Could you check a few things on this model? Use its own coordinates, in mm. Face numbers are marked on the shaded views. A direction names the side the tool comes from. Give positions to 0.01 mm unless a question says otherwise; leave off trailing zeros.
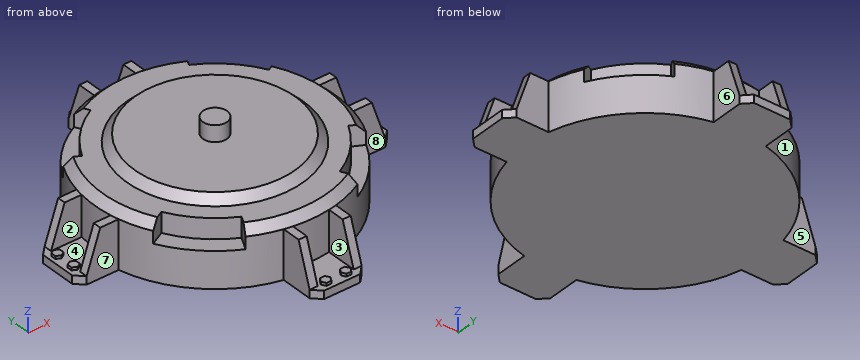
from build123d import *

# Parameters (mm, degrees)
SKETCH1_R                    = 150
BOSS_EXTRUDE1_DEPTH          = 70
CHAMFER1_SIZE                = 10
BOSS_EXTRUDE2_START          = -70
BOSS_EXTRUDE2_DEPTH          = 10
CHAMFER2_SIZE                = 10
BOSS_EXTRUDE3_DEPTH          = 10
BOSS_EXTRUDE4_DEPTH          = 3.5
CIRPATTERN1_COUNT            = 4
CIRPATTERN1_COPY_1_DEPTH     = 10
CIRPATTERN1_COPY_2_DEPTH     = 10
CIRPATTERN1_COPY_3_DEPTH     = 10
CIRPATTERN1_COPY_4_DEPTH     = 3.5
CIRPATTERN1_COPY_5_DEPTH     = 3.5
CIRPATTERN1_COPY_6_DEPTH     = 3.5
CHAMFER2_OF_CIRPATTERN1_SIZE = 10
CUT_EXTRUDE1_START           = -25
CUT_EXTRUDE1_DEPTH           = 25
CIRPATTERN2_COUNT            = 4
SKETCH6_R                    = 110
BOSS_EXTRUDE5_DEPTH          = 10
CHAMFER3_SIZE                = 10
SKETCH8_R                    = 15
BOSS_EXTRUDE6_DEPTH          = 20
BODY_MOVE_COPY2_ANGLE        = 90


with BuildPart() as part:
    # Sketch1 → Boss-Extrude1 (new body)
    with BuildSketch(Plane(origin=(0, 0, 0), x_dir=(1, 0, 0), z_dir=(0, 1, 0))):
        with Locations(Location((0, 0, 0), (0, 0, 270))):
            Circle(SKETCH1_R)
    extrude(amount=BOSS_EXTRUDE1_DEPTH)

    # Chamfer1
    chamfer1_edges = [part.edges().sort_by_distance(p)[0] for p in [
        (0, 70, -150),
    ]]
    chamfer(chamfer1_edges, length=CHAMFER1_SIZE)

    # Sketch2 → Boss-Extrude2 (add)
    with BuildSketch(Plane(origin=(0, 70, 0), x_dir=(1, 0, 0), z_dir=(0, 1, 0)).offset(BOSS_EXTRUDE2_START)):
        with BuildLine():
            Line((-146.436846456, 32.5), (-196.436846456, 32.5))
            Line((-196.436846456, 32.5), (-196.436846456, -32.5))
            Line((-196.436846456, -32.5), (-146.436846456, -32.5))
            ThreePointArc((-146.436846456, -32.5), (-150, 0), (-146.436846456, 32.5))
        make_face()
    boss_extrude2 = extrude(amount=BOSS_EXTRUDE2_DEPTH)

    # Chamfer2
    chamfer2_edges = [part.edges().sort_by_distance(p)[0] for p in [
        (-196.436846456, 5, -32.5),
        (-196.436846456, 5, 32.5),
    ]]
    chamfer(chamfer2_edges, length=CHAMFER2_SIZE)

    # Sketch3 → Boss-Extrude3 (add)
    with BuildSketch(Plane.XY.offset(32.5)):
        Polygon((-146.436846456, 10), (-146.436846456, 60), (-169.436846456, 60), (-186.436846456, 10), align=None)
    boss_extrude3 = extrude(amount=-BOSS_EXTRUDE3_DEPTH)

    # Sketch4 → Boss-Extrude4 (add)
    with BuildSketch(Plane(origin=(0, 10, 0), x_dir=(1, 0, 0), z_dir=(0, 1, 0))):
        Polygon((-186.436846456, -6.5), (-191.632998879, -9.5), (-191.632998879, -15.5), (-186.436846456, -18.5), (-181.240694033, -15.5), (-181.240694033, -9.5), align=None)
    boss_extrude4 = extrude(amount=BOSS_EXTRUDE4_DEPTH)

    # Mirror1: Boss-Extrude3, Boss-Extrude4 across plane
    add(boss_extrude3.mirror(Plane.XY))
    add(boss_extrude4.mirror(Plane.XY))

    # CirPattern1: Boss-Extrude2, Boss-Extrude3, Boss-Extrude4 ×4 about axis
    cirpattern1_axis = Axis((0, 0, 0), (0, 1, 0))
    add([boss_extrude2.rotate(cirpattern1_axis, i * 360 / CIRPATTERN1_COUNT) for i in range(1, CIRPATTERN1_COUNT)])
    add([boss_extrude3.rotate(cirpattern1_axis, i * 360 / CIRPATTERN1_COUNT) for i in range(1, CIRPATTERN1_COUNT)])
    add([boss_extrude4.rotate(cirpattern1_axis, i * 360 / CIRPATTERN1_COUNT) for i in range(1, CIRPATTERN1_COUNT)])

    # CirPattern1 copy 1 sketch → CirPattern1 copy 1 (add)
    with BuildSketch(Plane(origin=(-32.5, 0, 0), x_dir=(0, 0, -1), z_dir=(-1, 0, 0))):
        Polygon((-146.436846456, -10), (-146.436846456, -60), (-169.436846456, -60), (-186.436846456, -10), align=None)
    extrude(amount=-CIRPATTERN1_COPY_1_DEPTH)

    # CirPattern1 copy 2 sketch → CirPattern1 copy 2 (add)
    with BuildSketch(Plane(origin=(0, 0, 32.5), x_dir=(-1, 0, 0), z_dir=(0, 0, 1))):
        Polygon((-146.436846456, -10), (-146.436846456, -60), (-169.436846456, -60), (-186.436846456, -10), align=None)
    extrude(amount=-CIRPATTERN1_COPY_2_DEPTH)

    # CirPattern1 copy 3 sketch → CirPattern1 copy 3 (add)
    with BuildSketch(Plane(origin=(32.5, 0, 0), x_dir=(0, 0, 1), z_dir=(1, 0, 0))):
        Polygon((-146.436846456, -10), (-146.436846456, -60), (-169.436846456, -60), (-186.436846456, -10), align=None)
    extrude(amount=-CIRPATTERN1_COPY_3_DEPTH)

    # CirPattern1 copy 4 sketch → CirPattern1 copy 4 (add)
    with BuildSketch(Plane(origin=(0, 10, 0), x_dir=(0, 0, -1), z_dir=(0, 1, 0))):
        Polygon((-186.436846456, 6.5), (-191.632998879, 9.5), (-191.632998879, 15.5), (-186.436846456, 18.5), (-181.240694033, 15.5), (-181.240694033, 9.5), align=None)
    extrude(amount=CIRPATTERN1_COPY_4_DEPTH)

    # CirPattern1 copy 5 sketch → CirPattern1 copy 5 (add)
    with BuildSketch(Plane(origin=(0, 10, 0), x_dir=(-1, 0, 0), z_dir=(0, 1, 0))):
        Polygon((-186.436846456, 6.5), (-191.632998879, 9.5), (-191.632998879, 15.5), (-186.436846456, 18.5), (-181.240694033, 15.5), (-181.240694033, 9.5), align=None)
    extrude(amount=CIRPATTERN1_COPY_5_DEPTH)

    # CirPattern1 copy 6 sketch → CirPattern1 copy 6 (add)
    with BuildSketch(Plane.ZX.offset(10)):
        Polygon((-186.436846456, 6.5), (-191.632998879, 9.5), (-191.632998879, 15.5), (-186.436846456, 18.5), (-181.240694033, 15.5), (-181.240694033, 9.5), align=None)
    extrude(amount=CIRPATTERN1_COPY_6_DEPTH)

    # Chamfer2 of CirPattern1
    chamfer2_of_cirpattern1_edges = [part.edges().sort_by_distance(p)[0] for p in [
        (-32.5, 5, 196.436846456),
        (32.5, 5, 196.436846456),
        (196.436846456, 5, 32.5),
        (196.436846456, 5, -32.5),
        (32.5, 5, -196.436846456),
        (-32.5, 5, -196.436846456),
    ]]
    chamfer(chamfer2_of_cirpattern1_edges, length=CHAMFER2_OF_CIRPATTERN1_SIZE)

    # Sketch5 → Cut-Extrude1 (cut)
    with BuildSketch(Plane(origin=(0, 70, 0), x_dir=(1, 0, 0), z_dir=(0, 1, 0)).offset(CUT_EXTRUDE1_START)):
        with BuildLine():
            Line((-115.311408313, -60.027319721), (-133.051624977, -69.262291985))
            ThreePointArc((-133.051624977, -69.262291985), (-106.066017178, -106.066017178), (-69.262291985, -133.051624977))
            Line((-69.262291985, -133.051624977), (-60.027319721, -115.311408313))
            ThreePointArc((-60.027319721, -115.311408313), (-91.923881554, -91.923881554), (-115.311408313, -60.027319721))
        make_face()
    cut_extrude1 = extrude(amount=CUT_EXTRUDE1_DEPTH, mode=Mode.SUBTRACT)

    # CirPattern2: Cut-Extrude1 ×4 about axis
    cirpattern2_axis = Axis((1.276358498, 0, -1.276358498), (0, 1, 0))
    for i in range(1, CIRPATTERN2_COUNT):
        add(cut_extrude1.rotate(cirpattern2_axis, i * 360 / CIRPATTERN2_COUNT), mode=Mode.SUBTRACT)

    # Sketch6 → Boss-Extrude5 (add)
    with BuildSketch(Plane(origin=(0, 70, 0), x_dir=(1, 0, 0), z_dir=(0, 1, 0))):
        with Locations(Location((0, 0, 0), (0, 0, 270))):
            Circle(SKETCH6_R)
    extrude(amount=BOSS_EXTRUDE5_DEPTH)

    # Chamfer3
    chamfer3_edges = [part.edges().sort_by_distance(p)[0] for p in [
        (0, 80, -110),
    ]]
    chamfer(chamfer3_edges, length=CHAMFER3_SIZE - 0.0001)  # a hair under: the kernel refuses the full size

    # Sketch8 → Boss-Extrude6 (add)
    with BuildSketch(Plane(origin=(0, 80, 0), x_dir=(1, 0, 0), z_dir=(0, 1, 0))):
        with Locations(Location((0, 0, 0), (0, 0, 270))):
            Circle(SKETCH8_R)
    extrude(amount=BOSS_EXTRUDE6_DEPTH)


with BuildPart() as part_1:
    # Body-Move/Copy1: moved
    add(part.part.moved(Location((0, -99.99999995, 0))))


with BuildPart() as part_2:
    # Body-Move/Copy2: read off the stored shape, not the designer's step
    # Body-Move/Copy2: moved
    add(part_1.part.moved(Location((0, 50, 50))).rotate(Axis((0, 0, 0), (1, 0, 0)), BODY_MOVE_COPY2_ANGLE))


with BuildPart() as part_3:
    # Body-Move/Copy3: moved
    add(part_2.part.moved(Location((0, 50, -50))))


with BuildPart() as part_4:
    # Body-Move/Copy4: moved
    add(part_3.part.moved(Location((0, 0, 20))))


with BuildPart() as part_5:
    # Body-Move/Copy6: moved
    add(part_4.part.moved(Location((0, 0, 80))))


solid = part_5.part
Item 1: Please list where these lines run through material, in increasing order: line 1 along X through (y, z) = (-155.5, 40); line 2 along Z through (x, y) = (-97, 66); line 3 along Z through (x, y) = (35.5, -32).
Findings:
line 1: x = -32.5 to -22.5, 22.5 to 32.5
line 2: z = 0 to 70
line 3: z = 0 to 80
Item 2: We'd pull the mould along Y, two halves only. Please class the marked faces 1, 2, 3 and 4: +Y half, -Y half, draft (parallel to the pull), parting line (faces both ways), or undercut.
Findings:
face 1: +Y half
face 2: undercut
face 3: draft
face 4: undercut
Item 3: For pin 1 (8 mm diameter, centred on x = -92, z = 19.5, fed in from -Y); pin 2 (14.5 mm diameter, centred on x = 12.5, y = -174.5, fed in from +Z); pin 3 (5 mm diameter, centred on x = -161.5, y = 29, fed in from +Z), each with a flat end and sliding along its axis, tell me the tip position at first contact or that it passes through.
Findings:
pin 1: stops at y = -121.47
pin 2: stops at z = 13.5
pin 3: stops at z = 60
Item 4: For the marked faces 5, 6, 7 and 8, which set-ups out of +Z, -Z, +X, -X, +Y, -Y let a thin tool reach every point of the face, with its end or its side?
Findings:
face 5: +Z, -Z, -X, +Y
face 6: +Z, -Z, +X, +Y
face 7: +Z, -Z, -X, -Y
face 8: +Z, -Z, +X, -Y
